from build123d import *

# Parameters (mm, degrees)
F1_DEPTH = 95
F3_DEPTH = 10.001
F4_W     = 44.455645
F4_H     = 24.072581
F5_DEPTH = 61.3


with BuildPart() as f1:
    # F0 (on Right) → F1 (new body)
    with BuildSketch(Plane.YZ):
        Polygon((-60, 0), (0, 0), (0, 56), (-10, 56), (-10, 28), (-60, 13), align=None)
    extrude(amount=F1_DEPTH)

    # F2 (on face) → F3 (cut, through all)
    with BuildSketch(Plane.XZ.offset(10)):
        Polygon((95, 56), (57, 56), (95, 28), align=None)
    extrude(amount=-F3_DEPTH, mode=Mode.SUBTRACT)

    # F4 (on face) → F5 (cut)
    with BuildSketch(Plane(origin=(0, 0, 0), x_dir=(1, 0, 0), z_dir=(0, 0, -1))):
        with Locations((48.377015, 47.96371)):
            Rectangle(F4_W, F4_H)
    extrude(amount=-F5_DEPTH, mode=Mode.SUBTRACT)


solid = f1.part
Could you check a few things on this model? Use its own coordinates, in mm. A direction names the side the tool comes from. Give positions to 0.01 mm unless a question says otherwise; leave off trailing zeros. Order: outer loops, then holes, each group sorted by start corner. A loop starts at its lowest first (then second) coordinate and runs counter-clockwise, first axis right, second up. Notation, with made-up numbers: (28, 43.25) -> (35, 43.25) arc R14 ccw to (35, 68.25) -> close; hole circle Ø10 at (17.25, -11). An arc over 180 degrees is marked (long way). Return JSON: item names as keys, results as strings.
1. I need wall thicknesses on line 1 (Y direction, x = 29.5, z = 3.5); line 2 (Y direction, x = 47.5, z = 34); line 3 (X direction, y = -3, z = 45). Which ranges of each line are inside material? Lowest first, please. Write a range as from..to.
Answer list:
{"line 1": "y = -35.93..0", "line 2": "y = -10..0", "line 3": "x = 0..71.93"}
2. On a 3-axis mill with a long thin cutter (end or side, diameter ignored), from which of +Z, -Z, +X, -X, +Y, -Y can I reach the whole of each face in a straight line? I mean faces 1 (the flat face through (13, -60, 7)), 2 (the flat face through (36, -10, 42)), 3 (the flat face through (48, -35.927, 10)). Say none if no direction works.
Answer list:
{"face 1": "+Z, -Z, +X, -X, -Y", "face 2": "+Z, +X, -X, -Y", "face 3": "+Z, -Z, -Y"}
3. Thinking about a two-plate mould opening in X: for faces 4 (the flat face through (47, -24, 0)), 5 (the flat face through (76, -5, 42)), 6 (the flat face through (26.149, -48, 8)), which applies, pulls with the +X half, pulls with the -X half, needs draft (parallel to the pull), parting line crosses it, or undercut?
Answer list:
{"face 4": "needs draft", "face 5": "pulls with the +X half", "face 6": "undercut"}
4. Imagine slicing it at C-C on z = 3. List the corners of the cut face in (x, y) for me, then the cut area to 3 significant figures.
Answer list:
{"outline": "(0, -60) -> (26.15, -60) -> (26.15, -35.93) -> (70.6, -35.93) -> (70.6, -60) -> (95, -60) -> (95, 0) -> (0, 0) -> close", "area": "4,630 mm2"}
5. Imagine slicing it at A-A on y = -49.5. List the corners of the cut face in (x, z) for me.
Answer list:
{"outline": "(0, 0) -> (26.15, 0) -> (26.15, 16.15) -> (0, 16.15) -> close; (70.6, 0) -> (95, 0) -> (95, 16.15) -> (70.6, 16.15) -> close"}
6. Imagine slicing it at B-B on x = 55. List the corners of the cut face in (y, z) for me.
Answer list:
{"outline": "(-35.93, 0) -> (0, 0) -> (0, 56) -> (-10, 56) -> (-10, 28) -> (-35.93, 20.22) -> close"}
7. For pin 1 Ø14 at (x, z) = (40, 41.5) entering from -Y; pin 2 Ø12 at (x, z) = (61.5, 15) entering from -Y; pin 3 Ø1 at (y, z) = (-11, 36) entering from +X, each with a flat end and sliding along its axis, tell me the tip position at first contact or that it passes through.
Answer list:
{"pin 1": "stops at y = -10", "pin 2": "stops at y = -35.93", "pin 3": "passes through"}
8. Imagine slicing it at D-D on y = -43. List the corners of the cut face in (x, z) for me, then the cut area to 3 significant figures.
Answer list:
{"outline": "(0, 0) -> (26.15, 0) -> (26.15, 18.1) -> (0, 18.1) -> close; (70.6, 0) -> (95, 0) -> (95, 18.1) -> (70.6, 18.1) -> close", "area": "915 mm2"}
